Check sheet for the drawn part. Datum: minimum x, y, z corner. Units: mm. A direction names the side the tool comes from. Round coordinates to 2 decimals unless told otherwise and drop trailing zeros. Order: outer loops, then holes, each group sorted by start corner. A loop starts at its lowest first (then second) coordinate and runs counter-clockwise, first axis right, second up. Notation, with made-up numbers: (-38, 4) -> (-10, 4) arc R8 cw to (-10, 11) -> close; hole circle Ø1 at (15, -8.5). An arc over 180 degrees is marked (long way). Write item = value, one per line. Start each with the question number.
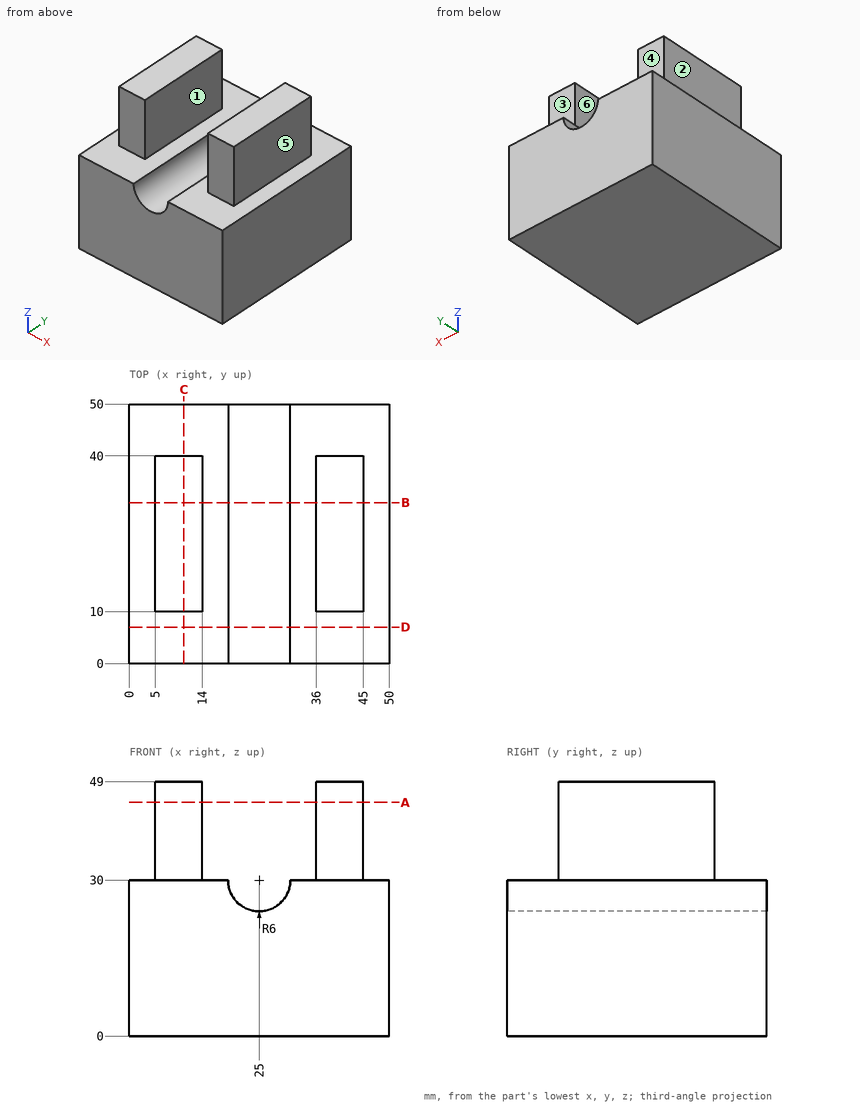
(1) Cross-section at B-B (y = 31). Enter the section's corners in (x, z).
(2) Cross-section at D-D (y = 7). Enter the section's corners in (x, z), and give its area (3 significant figures).
(3) Draft check along X on the marked faces 4, 5 and 6. Enter one of: +X half, -X half, draft (parallel to the pull), parting line (faces both ways), or undercut.
(4) Depth check by flat-ended pin: pin 1 (10 mm diameter, centred on x = 9.5, z = 40, fed in from -Y); pin 2 (8 mm diameter, centred on x = 25.5, y = 19, fed in from +Z); pin 3 (4.5 mm diameter, centred on x = 40, z = 42, fed in from +Y). Enter the tip coordinate at first touch or a pass-through.
(5) Cross-section at A-A (z = 45). Enter the section's corners in (x, y), and give its area (3 significant figures).
(6) Cross-section at C-C (x = 10.5). Enter the section's corners in (y, z), and give its area (3 significant figures).
(7) Set-up check for the marked faces 1, 2 and 3: record each of +Z, -Z, +X, -X, +Y, -Y from which the full face is reachable in a straight line by a thin tool's end or side.
(8) Scan lines: line 1 along X through (y, z) = (13, 39); line 2 along Z through (x, y) = (33.5, 10.5); line 3 along X through (y, z) = (33.5, 25.5). Record each from-to range of solid material in increasing order. Write a range as from..to.
Outcome:
q1.outline = (0, 0) -> (50, 0) -> (50, 30) -> (45, 30) -> (45, 49) -> (36, 49) -> (36, 30) -> (31, 30) arc R6 cw to (19, 30) -> (14, 30) -> (14, 49) -> (5, 49) -> (5, 30) -> (0, 30) -> close
q2.outline = (0, 0) -> (50, 0) -> (50, 30) -> (31, 30) arc R6 cw to (19, 30) -> (0, 30) -> close
q2.area = 1,440 mm^2
q3.face_4 = draft
q3.face_5 = +X half
q3.face_6 = undercut
q4.pin_1 = 10
q4.pin_2 = 26.03
q4.pin_3 = 40
q5.outline = (5, 10) -> (14, 10) -> (14, 40) -> (5, 40) -> close; (36, 10) -> (45, 10) -> (45, 40) -> (36, 40) -> close
q5.area = 540 mm^2
q6.outline = (0, 0) -> (50, 0) -> (50, 30) -> (40, 30) -> (40, 49) -> (10, 49) -> (10, 30) -> (0, 30) -> close
q6.area = 2,070 mm^2
q7.face_1 = +Z, +Y, -Y
q7.face_2 = +Z, -X, +Y, -Y
q7.face_3 = +Z, +X, -X, +Y
q8.line_1 = 5..14, 36..45
q8.line_2 = 0..30
q8.line_3 = 0..21.03, 28.97..50
